The model under review builds one solid part; all positions refer to its coordinate system, in mm. A direction names the side the tool comes from. Round coordinates to 2 decimals unless told otherwise and drop trailing zeros. Loops run counter-clockwise (first coordinate to the right, second up) from the corner with the lowest first, then second, coordinate; pieces in that order, holes last. Notation, with made-up numbers: (84, 31.25) -> (128, 31.25) arc R8 ccw to (128, 42.25) -> close; hole circle Ø11 at (3.25, 44). An arc over 180 degrees is marked (long way). Use CSV: the item, a comma, the result in double quotes. Start each with the question number.
```python
from build123d import *

# Parameters (mm, degrees)
BASEPLATE_OUTLINE_R = 2.1
BASEPLATE_DEPTH     = 2.8
CUT_EXTRUDE1_REACH  = 115.438
SKETCH3_W           = 15.4
SKETCH3_H           = 19.2
SKETCH3_W_2         = 15.6
SKETCH3_W_3         = 16.2
SKETCH3_H_2         = 24.9
CUT_EXTRUDE2_REACH  = 115.438
SKETCH4_W           = 2
SKETCH4_H           = 10.2
FILLET1_R           = 5


# Read off the part's stored shape, not the designer's step: BasePlate
with BuildPart() as part:
    # BasePlate outline → BasePlate (new body)
    with BuildSketch(Plane(origin=(0, 0, 0), x_dir=(1, 0, 0), z_dir=(0, 1, 0))):
        with BuildLine():
            Line((43.502626614, -5.852332608), (48.792614178, -5.852332608))
            ThreePointArc((48.792614178, -5.852332608), (49.082078508, -5.760021707), (49.264659986, -5.517174213))
            Line((49.264659986, -5.517174213), (50.078201202, -3.187491002))
            ThreePointArc((50.078201202, -3.187491002), (50.26078268, -2.944643509), (50.55024701, -2.852332608))
            Line((50.55024701, -2.852332608), (58.116695703, -2.852332608))
            ThreePointArc((58.116695703, -2.852332608), (58.484685739, -3.013831008), (58.614956567, -3.393999275))
            ThreePointArc((58.614956567, -3.393999275), (64.799237397, -7.61016844), (65.229166667, -0.137781095))
            ThreePointArc((65.229166667, -0.137781095), (65.061014427, 0.043158816), (65, 0.282515593))
            Line((65, 0.282515593), (65, 83.012819192))
            ThreePointArc((65, 83.012819192), (65.061014427, 83.252175969), (65.229166667, 83.433115879))
            ThreePointArc((65.229166667, 83.433115879), (65.940559159, 90.088226551), (59.285448487, 89.376834059))
            ThreePointArc((59.285448487, 89.376834059), (59.104508577, 89.208681819), (58.8651518, 89.147667392))
            Line((58.8651518, 89.147667392), (6.1348482, 89.147667392))
            ThreePointArc((6.1348482, 89.147667392), (5.895491423, 89.208681819), (5.714551513, 89.376834059))
            ThreePointArc((5.714551513, 89.376834059), (-0.940559159, 90.088226551), (-0.229166667, 83.433115879))
            ThreePointArc((-0.229166667, 83.433115879), (-0.061014427, 83.252175969), (0, 83.012819192))
            Line((0, 83.012819192), (0, 0.282515593))
            ThreePointArc((0, 0.282515593), (-0.061014427, 0.043158816), (-0.229166667, -0.137781095))
            ThreePointArc((-0.229166667, -0.137781095), (0.200762603, -7.61016844), (6.385043433, -3.393999275))
            ThreePointArc((6.385043433, -3.393999275), (6.515314261, -3.013831008), (6.883304297, -2.852332608))
            Line((6.883304297, -2.852332608), (14.44975299, -2.852332608))
            ThreePointArc((14.44975299, -2.852332608), (14.73921732, -2.944643509), (14.921798798, -3.187491002))
            Line((14.921798798, -3.187491002), (15.735340014, -5.517174213))
            ThreePointArc((15.735340014, -5.517174213), (15.917921492, -5.760021707), (16.207385822, -5.852332608))
            Line((16.207385822, -5.852332608), (21.497373386, -5.852332608))
            ThreePointArc((21.497373386, -5.852332608), (21.786837716, -5.760021707), (21.969419194, -5.517174213))
            Line((21.969419194, -5.517174213), (22.78296041, -3.187491002))
            ThreePointArc((22.78296041, -3.187491002), (22.965541888, -2.944643509), (23.255006218, -2.852332608))
            Line((23.255006218, -2.852332608), (41.744993782, -2.852332608))
            ThreePointArc((41.744993782, -2.852332608), (42.034458112, -2.944643509), (42.21703959, -3.187491002))
            Line((42.21703959, -3.187491002), (43.030580806, -5.517174213))
            ThreePointArc((43.030580806, -5.517174213), (43.213162284, -5.760021707), (43.502626614, -5.852332608))
        make_face()
        with Locations((2.1, -3.752332608)):
            Circle(BASEPLATE_OUTLINE_R, mode=Mode.SUBTRACT)
        with Locations((62.9, -3.752332608)):
            Circle(BASEPLATE_OUTLINE_R, mode=Mode.SUBTRACT)
        with Locations((2.1, 87.047667392)):
            Circle(BASEPLATE_OUTLINE_R, mode=Mode.SUBTRACT)
        with Locations((62.9, 87.047667392)):
            Circle(BASEPLATE_OUTLINE_R, mode=Mode.SUBTRACT)
    extrude(amount=BASEPLATE_DEPTH)

    # Sketch3 → Cut-Extrude1 (cut, up to next)
    with BuildSketch(Plane(origin=(0, 2.8, 0), x_dir=(1, 0, 0), z_dir=(0, 1, 0)), mode=Mode.PRIVATE) as cut_extrude1_sk1:
        Polygon((4.8, 1.147667392), (49.5, 1.147667392), (49.5, 24.447667392), (63, 24.447667392), (63, 22.647667392), (65, 22.647667392), (65, 42.047667392), (63, 42.047667392), (63, 40.047667392), (35.4, 40.047667392), (35.4, 61.647667392), (33.1, 61.647667392), (33.1, 66.147667392), (19.8, 66.147667392), (19.8, 61.647667392), (4.8, 61.647667392), align=None)
    cut_extrude1_tool1 = extrude(cut_extrude1_sk1.sketch, amount=-CUT_EXTRUDE1_REACH, mode=Mode.PRIVATE) & part.part
    # Sketch3 → Cut-Extrude1 (cut, up to next)
    with BuildSketch(Plane(origin=(0, 2.8, 0), x_dir=(1, 0, 0), z_dir=(0, 1, 0)), mode=Mode.PRIVATE) as cut_extrude1_sk2:
        with Locations((14, 79.547667392)):
            Rectangle(SKETCH3_W, SKETCH3_H)
    cut_extrude1_tool2 = extrude(cut_extrude1_sk2.sketch, amount=-CUT_EXTRUDE1_REACH, mode=Mode.PRIVATE) & part.part
    # Sketch3 → Cut-Extrude1 (cut, up to next)
    with BuildSketch(Plane(origin=(0, 2.8, 0), x_dir=(1, 0, 0), z_dir=(0, 1, 0)), mode=Mode.PRIVATE) as cut_extrude1_sk3:
        with Locations((32, 79.547667392)):
            Rectangle(SKETCH3_W_2, SKETCH3_H)
    cut_extrude1_tool3 = extrude(cut_extrude1_sk3.sketch, amount=-CUT_EXTRUDE1_REACH, mode=Mode.PRIVATE) & part.part
    # Sketch3 → Cut-Extrude1 (cut, up to next)
    with BuildSketch(Plane(origin=(0, 2.8, 0), x_dir=(1, 0, 0), z_dir=(0, 1, 0)), mode=Mode.PRIVATE) as cut_extrude1_sk4:
        with Locations((51, 76.697667392)):
            Rectangle(SKETCH3_W_3, SKETCH3_H_2)
    cut_extrude1_tool4 = extrude(cut_extrude1_sk4.sketch, amount=-CUT_EXTRUDE1_REACH, mode=Mode.PRIVATE) & part.part
    add(cut_extrude1_tool1.solids().sort_by_distance((28.204461, 2.8, -30.008726))[0], mode=Mode.SUBTRACT)
    add(cut_extrude1_tool2.solids().sort_by_distance((14, 2.8, -79.547667))[0], mode=Mode.SUBTRACT)
    add(cut_extrude1_tool3.solids().sort_by_distance((32, 2.8, -79.547667))[0], mode=Mode.SUBTRACT)
    add(cut_extrude1_tool4.solids().sort_by_distance((51, 2.8, -76.697667))[0], mode=Mode.SUBTRACT)

    # Sketch4 → Cut-Extrude2 (cut, up to next)
    with BuildSketch(Plane(origin=(0, 2.8, 0), x_dir=(1, 0, 0), z_dir=(0, 1, 0)), mode=Mode.PRIVATE) as cut_extrude2_sk1:
        with Locations((64, 53.147667392)):
            Rectangle(SKETCH4_W, SKETCH4_H)
    cut_extrude2_tool1 = extrude(cut_extrude2_sk1.sketch, amount=-CUT_EXTRUDE2_REACH, mode=Mode.PRIVATE) & part.part
    # Sketch4 → Cut-Extrude2 (cut, up to next)
    with BuildSketch(Plane(origin=(0, 2.8, 0), x_dir=(1, 0, 0), z_dir=(0, 1, 0)), mode=Mode.PRIVATE) as cut_extrude2_sk2:
        Polygon((60.9, 56.247667392), (40.2, 56.247667392), (40.2, 47.947667392), (38.3, 47.947667392), (38.3, 42.447667392), (60.9, 42.447667392), (60.9, 50.047667392), align=None)
    cut_extrude2_tool2 = extrude(cut_extrude2_sk2.sketch, amount=-CUT_EXTRUDE2_REACH, mode=Mode.PRIVATE) & part.part
    add(cut_extrude2_tool1.solids().sort_by_distance((64, 2.8, -53.147667))[0], mode=Mode.SUBTRACT)
    add(cut_extrude2_tool2.solids().sort_by_distance((50.151212, 2.8, -49.20121))[0], mode=Mode.SUBTRACT)

    # Fillet1
    fillet1_edges = [part.edges().sort_by_distance(p)[0] for p in [
        (49.5, 1.4, -24.447667392),
    ]]
    fillet(fillet1_edges, radius=FILLET1_R)


solid = part.part
```
1. Take a section at A-A, the plane x = 2.1. Give the boundary of the cut face in (y, z), then the cut area to 3 significant figures.
2. For line 1 along X through (y, z) = (1.3, -44.5); line 2 along X through (y, z) = (1.55, -65); line 3 along Z through (x, y) = (62.9, 0.7), list the stretches that pass through material, from the lowest coordinate up. Write a range as from..to.
3. Clearance check with flat-ended pins moving along their axes: P1, Ø0.6, axis at x = 63.5, y = 2, coming from the +Z side; P2, Ø1.6, axis at x = 64.5, y = 1, coming from the -Z side; P3, Ø1.4, axis at y = 0.5, z = -23, coming from the +X side; P4, Ø2.5, axis at x = 2.1, z = -87.05, coming from the +Y side. State where each tip first meets the part, or that it passes through.
4. The part is to be moulded in two halves that separate along Z. For faces 5 (the face through (40, 2.8, -42)), 6 (the face through (54, 1, 2.852)), 7 (the face through (65, 1, -11)), say which applies: pulls with the +Z half, pulls with the -Z half, needs draft (parallel to the pull), parting line crosses it, or undercut.
5. Take a section at D-D, the plane z = -11.5. Give the boundary of the cut face in (x, y), then the cut area to 3 significant figures.
6. Take a section at C-C, the plane x = 29. Give the boundary of the cut face in (y, z), then the cut area to 3 significant figures.
7. Take a section at B-B, the plane z = -53.5. Give the boundary of the cut face in (x, y), then the cut area to 3 significant figures.
8. For faces 1 (the face through (11, 1, 2.852)), 2 (the face through (64, 1, -42.048)), 3 (the face through (38.3, 1, -45)), 4 (the face through (41, 1, -89.148)), list the 3-axis set-ups (+Z, -Z, +X, -X, +Y, -Y) from which the entire face can be reached by the end or side of a thin tool; tool diameter is ignored.
Results:
1,outline,"(0, -91.35) -> (2.8, -91.35) -> (2.8, -89.15) -> (0, -89.15) -> close; (0, -84.95) -> (2.8, -84.95) -> (2.8, 1.65) -> (0, 1.65) -> close; (0, 5.85) -> (2.8, 5.85) -> (2.8, 8.05) -> (0, 8.05) -> close"
1,area,"255 mm²"
2,line 1,"0..4.8, 35.4..38.3, 60.9..65"
2,line 2,"0..19.8, 33.1..42.9, 59.1..65"
2,line 3,"-91.35..-89.15, -84.95..-40.05, -24.45..1.65, 5.85..8.05"
3,P1,"z = 8.04"
3,P2,"z = -91.27"
3,P3,"x = 65"
3,P4,"through"
4,face 5,"needs draft"
4,face 6,"pulls with the +Z half"
4,face 7,"undercut"
5,outline,"(0, 0) -> (4.8, 0) -> (4.8, 2.8) -> (0, 2.8) -> close; (49.5, 0) -> (65, 0) -> (65, 2.8) -> (49.5, 2.8) -> close"
5,area,"56.8 mm²"
6,outline,"(0, -69.95) -> (2.8, -69.95) -> (2.8, -66.15) -> (0, -66.15) -> close; (0, -1.15) -> (2.8, -1.15) -> (2.8, 2.85) -> (0, 2.85) -> close"
6,area,"21.8 mm²"
7,outline,"(0, 0) -> (4.8, 0) -> (4.8, 2.8) -> (0, 2.8) -> close; (35.4, 0) -> (40.2, 0) -> (40.2, 2.8) -> (35.4, 2.8) -> close; (60.9, 0) -> (63, 0) -> (63, 2.8) -> (60.9, 2.8) -> close"
7,area,"32.8 mm²"
8,face 1,"+Z, +Y, -Y"
8,face 2,"+X, +Y, -Y"
8,face 3,"+Y, -Y"
8,face 4,"-Z, +Y, -Y"
